Job drawing, mm, ordinate dimensions from the low corner. One solid piece. Coordinates: 2 decimals unless noted, no trailing zeros. Write each loop counter-clockwise with the first axis right and the second up, starting at its lowest first coordinate (ties: lowest second). Pieces come first, ordered by that corner, then holes. Notation, with made-up numbers: (18.5, 0.25) - (72.5, 0.25) arc R20 ccw to (72.5, 11.25) - close; hole circle Ø9 at (79, -11.5). An arc over 180 degrees is marked (long way). Use a Markdown table: item, result.
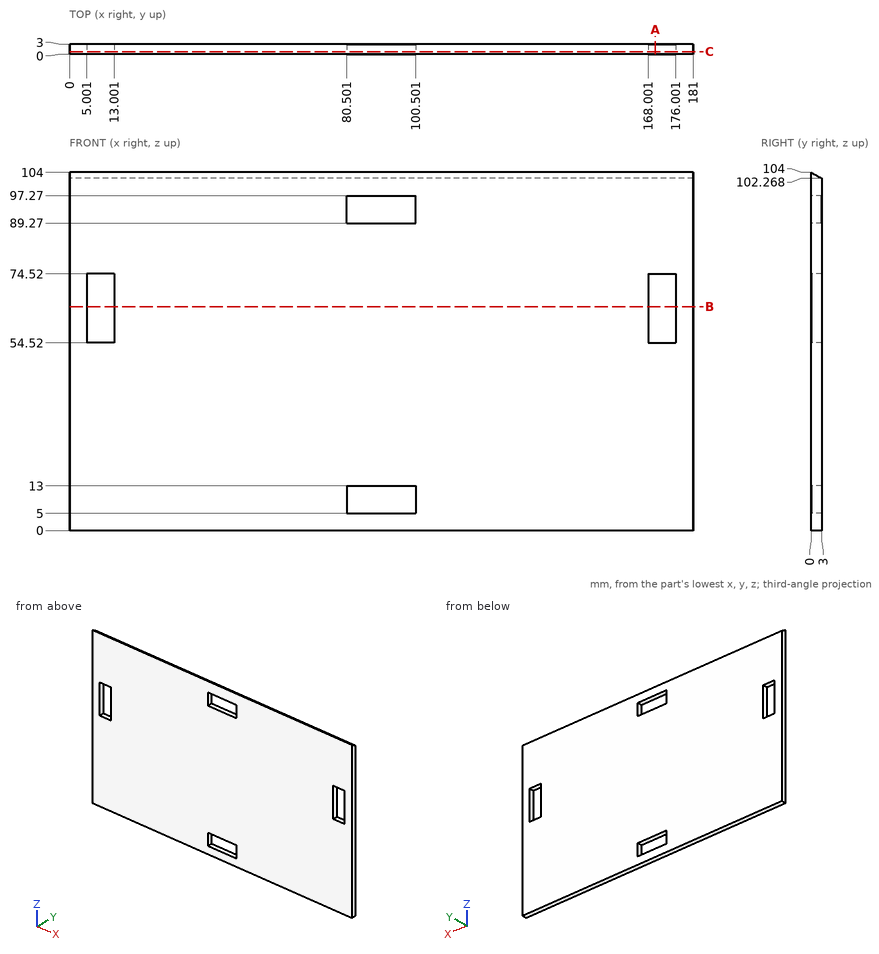
Item 1: Band-saw the part on B-B, the plane z = 65. Give the cut face in (x, y), then the cut area to 3 significant figures.
From the geometry:
| item | result |
|---|---|
| outline | (0, 0) - (5, 0) - (5, 3) - (0, 3) - close; (13, 0) - (168, 0) - (168, 3) - (13, 3) - close; (176, 0) - (181, 0) - (181, 3) - (176, 3) - close |
| area | 495 mm^2 |
Item 2: Drop flat-ended pins along their axis: P1, Ø1.5, axis at x = 92, y = 1, coming from the +Z side (1 decimal); P2, Ø1.5, axis at x = 91.5, y = 2, coming from the +Z side; P3, Ø1, axis at x = 119, y = 1.5, coming from the +Z side. Give the stop position or say it passes through.
From the geometry:
| item | result |
|---|---|
| P1 | z = 103.9 |
| P2 | z = 103.28 |
| P3 | z = 103.42 |
Item 3: Band-saw the part on C-C, the plane y = 0.75. Give the cut face in (x, z).
From the geometry:
| item | result |
|---|---|
| outline | (0, 0) - (181, 0) - (181, 103.57) - (0, 103.57) - close; hole (5, 54.52) - (13, 54.52) - (13, 74.52) - (5, 74.52) - close; hole (80.5, 5) - (100.5, 5) - (100.5, 13) - (80.5, 13) - close; hole (80.5, 89.27) - (100.5, 89.27) - (100.5, 97.27) - (80.5, 97.27) - close; hole (168, 54.52) - (176, 54.52) - (176, 74.52) - (168, 74.52) - close |
Item 4: Band-saw the part on A-A, the plane x = 170. Give the cut face in (y, z), then the cut area to 3 significant figures.
From the geometry:
| item | result |
|---|---|
| outline | (0, 0) - (3, 0) - (3, 54.52) - (0, 54.52) - close; (0, 74.52) - (3, 74.52) - (3, 102.27) - (0, 104) - close |
| area | 249 mm^2 |
Item 5: Drill centre lines: probe 1 along X at (y, z) = (1.2, 67); probe 2 along Z at (x, y) = (94.5, 1); probe 3 along Z at (x, y) = (95, 1.8). Where is each one in solid material? Low to high.
From the geometry:
| item | result |
|---|---|
| probe 1 | 0 to 5, 13 to 168, 176 to 181 |
| probe 2 | 0 to 5, 13 to 89.27, 97.27 to 103.42 |
| probe 3 | 0 to 5, 13 to 89.27, 97.27 to 102.96 |
